```python
from build123d import *

# Parameters (mm, degrees)
BOSS_EXTRUDE1_DEPTH     = 300.25
SKETCH3_W               = 20
SKETCH3_H               = 20
CUT_EXTRUDE1_DEPTH      = 1040.5
CUT_EXTRUDE2_DEPTH      = 303.20069904
CUT_EXTRUDE2_DEPTH_BACK = 303.20069904


with BuildPart() as part:
    # Sketch1 → Boss-Extrude1 (new body)
    with BuildSketch(Plane(origin=(0, 0, 0), x_dir=(1, 0, 0), z_dir=(0, 1, 0))):
        with BuildLine():
            Line((2.8, 0), (22.8, 0))
            ThreePointArc((22.8, 0), (24.779898987, -0.820101013), (25.6, -2.8))
            Line((25.6, -2.8), (25.6, -22.8))
            ThreePointArc((25.6, -22.8), (24.779898987, -24.779898987), (22.8, -25.6))
            Line((22.8, -25.6), (2.8, -25.6))
            ThreePointArc((2.8, -25.6), (0.820101013, -24.779898987), (0, -22.8))
            Line((0, -22.8), (0, -2.8))
            ThreePointArc((0, -2.8), (0.820101013, -0.820101013), (2.8, 0))
        make_face()
    extrude(amount=BOSS_EXTRUDE1_DEPTH)

    # Sketch3 → Cut-Extrude1 (cut)
    with BuildSketch(Plane(origin=(0, 0, 0), x_dir=(-1, 0, 0), z_dir=(0, -1, 0))):
        with Locations((-12.8, -12.8)):
            Rectangle(SKETCH3_W, SKETCH3_H)
    extrude(amount=-CUT_EXTRUDE1_DEPTH, mode=Mode.SUBTRACT)

    # Sketch4 → Cut-Extrude2 (cut, two sides: drawn at the far end of the back side and taken through both)
    with BuildSketch(Plane.XY.offset(22.8).offset(-CUT_EXTRUDE2_DEPTH_BACK)):
        Polygon((-582.227773903, 491.001368364), (0, 300.25), (25.6, 291.862844236), (607.827773903, 101.111475872), (989.330510631, 1265.567023678), (-200.725037175, 1655.456916171), align=None)
    extrude(amount=CUT_EXTRUDE2_DEPTH + CUT_EXTRUDE2_DEPTH_BACK, mode=Mode.SUBTRACT)


solid = part.part
```
Geometry check sheet. Reference: the model listing, model coordinates, mm. A direction names the side the tool comes from. Round coordinates to 2 decimals unless told otherwise and drop trailing zeros. Order: outer loops, then holes, each group sorted by start corner. A loop starts at its lowest first (then second) coordinate and runs counter-clockwise, first axis right, second up. Notation, with made-up numbers: (12, 25) - (36, 25) arc R32 ccw to (36, 59) - close; hole circle Ø3 at (43, 54.5). An arc over 180 degrees is marked (long way). Use a Markdown table: item, result. Add a question column.
1) Thickness scan on line 1 along X through (y, z) = (72, 16); line 2 along X through (y, z) = (33, 2.5). Record the ranges inside material, lowest first.
2) Section check C-C (y = 67). Record the cut outline in (x, z), then the cut area to 3 significant figures.
3) Mould release check, pull along Z, two halves, no side actions. Record for faces 1 (the flat face through (2.8, 148, 13)), 2 (the flat face through (13, 148, 25.6)), 3 (the flat face through (2, 0, 13)): released by +Z, released by -Z, zero draft, split by the parting line, or undercut.
4) Section check A-A (z = 15.5). Record the cut outline in (x, y), then the cut area to 3 significant figures.
5) Gauge pin test, flat ends, axial feed: P1, Ø1.5, axis at x = 16, z = 4, coming from the -Y side; P2, Ø4, axis at x = 22, z = 20.5, coming from the +Y side. Record the tip position at first contact, or that the pin passes through.
6) Section check B-B (x = 20). Record the cut outline in (y, z).
7) Set-up check for faces 4 (the flat face through (13, 148, 2.8)), 5 (the flat face through (0, 148, 13)): record each of +Z, -Z, +X, -X, +Y, -Y from which the full face is reachable in a straight line by a thin tool's end or side.
Established:
| question | item | result |
|---|---|---|
| 1 | line 1 | 0 to 2.8, 22.8 to 25.6 |
| 1 | line 2 | 0.02 to 25.58 |
| 2 | outline | (0, 2.8) arc R2.8 ccw to (2.8, 0) - (22.8, 0) arc R2.8 ccw to (25.6, 2.8) - (25.6, 22.8) arc R2.8 ccw to (22.8, 25.6) - (2.8, 25.6) arc R2.8 ccw to (0, 22.8) - close; hole (2.8, 2.8) - (22.8, 2.8) - (22.8, 22.8) - (2.8, 22.8) - close |
| 2 | area | 249 mm2 |
| 3 | face 1 | undercut |
| 3 | face 2 | released by +Z |
| 3 | face 3 | zero draft |
| 4 | outline | (0, 0) - (2.8, 0) - (2.8, 299.33) - (0, 300.25) - close; (22.8, 0) - (25.6, 0) - (25.6, 291.86) - (22.8, 292.78) - close |
| 4 | area | 1,660 mm2 |
| 5 | P1 | through |
| 5 | P2 | y = 292.78 |
| 6 | outline | (0, 0) - (293.7, 0) - (293.7, 2.8) - (0, 2.8) - close; (0, 22.8) - (293.7, 22.8) - (293.7, 25.6) - (0, 25.6) - close |
| 7 | face 4 | +Y, -Y |
| 7 | face 5 | +Z, -Z, -X, +Y, -Y |
